from build123d import *

# Parameters (mm, degrees)
F0_W           = 430
F0_H           = 100
F1_DEPTH       = 10
F3_D           = 17.5
F4_D           = 5
F4_CBORE_D     = 11.25
F4_CBORE_DEPTH = 6
F5_D           = 6
F8_R           = 10
F9_DEPTH       = 10


with BuildPart() as f1:
    # F0 (on Front) → F1 (new body)
    with BuildSketch(Plane.XZ):
        with Locations((215, 50)):
            Rectangle(F0_W, F0_H)
    extrude(amount=F1_DEPTH)

    # F3 (through all)
    with Locations(Plane.XZ.offset(10)):
        with Locations((47.26, 57.03), (159.02, 57.03), (270.78, 57.03), (382.54, 57.03)):
            Hole(F3_D / 2)

    # F4 (through all)
    with Locations(Plane.XZ.offset(10)):
        with Locations((10, 90), (112.5, 90), (215, 90), (317.5, 90), (420, 90), (420, 10), (317.5, 10), (215, 10), (112.05, 10), (10, 10)):
            CounterBoreHole(F4_D / 2, F4_CBORE_D / 2, F4_CBORE_DEPTH)

    # F5 (through all)
    with Locations(Plane.XZ.offset(10)):
        with Locations((10, 50), (215, 50), (420, 50)):
            Hole(F5_D / 2)

    # F8 (on line) → F9 (cut)
    with BuildSketch(Plane(origin=(0, -24.8257901338, 20.831311345), x_dir=(-1, 0, 0), z_dir=(0, 0.7660444431, -0.6427876097))):
        with Locations((-16.1151010543, 22.157035768)):
            Circle(F8_R)
        with Locations((-81.1700448394, 22.157035768)):
            Circle(F8_R)
        with Locations((-175.6755411625, 22.157035768)):
            Circle(F8_R)
        with Locations((-295.1289117336, 22.157035768)):
            Circle(F8_R)
        with Locations((-396.9926536083, 22.157035768)):
            Circle(F8_R)
    extrude(amount=-F9_DEPTH, mode=Mode.SUBTRACT)


solid = f1.part
Input: part model. Units: mm. Frame: model coordinates. A direction names the side the tool comes from. Give positions to 0.01 mm unless a question says otherwise; leave off trailing zeros. Loops run counter-clockwise (first coordinate to the right, second up) from the corner with the lowest first, then second, coordinate; pieces in that order, holes last. Notation, with made-up numbers: (89, 69) -> (102, 69) arc R5 cw to (102, 77) -> close; hole circle Ø11 at (13.5, 85). An arc over 180 degrees is marked (long way). Answer as a JSON object with one key per item and string values. Group by question number.
Item 1: Pin query (flat end, axial travel): P1, Ø5.5, axis at x = 216, z = 10.5, coming from the -Y side; P2, Ø10.5, axis at x = 47.26, z = 57.03, coming from the +Y side. Return the tip coordinate at first contact, or that it passes through.
Item 2: Cut plane B-B, the plane z = 57.03. Return the cut outline in (x, y).
Item 3: Pull-direction query (X, two-part tool) for faces 3 (the flat face through (430, -5, 49)), 4 (the flat face through (216.2, -4, 87.6)), 5 (the flat face through (212, 0, 51)); classes: released by +X, released by -X, zero draft, split by the parting line, or undercut.
Item 4: Line query: probe 1 along Z at (x, y) = (420, -1.8); probe 2 along Z at (x, y) = (47.26, -7); probe 3 along X at (y, z) = (-6.75, 86). Output: solid intervals per line, ascending.
Item 5: Cut plane A-A, the plane x = 47.26. Return the cut outline in (y, z).
Item 6: Cut plane C-C, the plane x = 292.5. Return the cut outline in (y, z).
Item 7: Reachability of faces 1 (the cylindrical face through (39.177, -4.93, 53.679)), 2 (the flat face through (295.268, -7.686, 41.257)) from +Z, -Z, +X, -X, +Y, -Y: full face, straight path, thin tool, end or side. Return the list, or none.
Item 8: Cut plane D-D, the plane y = -6.75. State how many separate pieces and enclosed holes the cut face has, and give its area (3 significant figures).
Checks:
{
 "1": {"P1": "stops at y = -4", "P2": "passes through"},
 "2": {"outline": "(0, -10) -> (38.51, -10) -> (38.51, 0) -> (0, 0) -> close; (56.01, -10) -> (150.27, -10) -> (150.27, 0) -> (56.01, 0) -> close; (167.77, -10) -> (262.03, -10) -> (262.03, 0) -> (167.77, 0) -> close; (279.53, -10) -> (373.79, -10) -> (373.79, 0) -> (279.53, 0) -> close; (391.29, -10) -> (430, -10) -> (430, 0) -> (391.29, 0) -> close"},
 "3": {"face 3": "released by +X", "face 4": "undercut", "face 5": "zero draft"},
 "4": {"probe 1": "z = 0 to 7.5, 12.5 to 47, 53 to 87.5, 92.5 to 100", "probe 2": "z = 0 to 48.28, 65.78 to 100", "probe 3": "x = 0 to 6.05, 13.95 to 108.55, 116.45 to 211.05, 218.95 to 313.55, 321.45 to 416.05, 423.95 to 430"},
 "5": {"outline": "(-10, 0) -> (0, 0) -> (0, 48.28) -> (-10, 48.28) -> close; (-10, 65.78) -> (0, 65.78) -> (0, 100) -> (-10, 100) -> close"},
 "6": {"outline": "(-10, 0) -> (0, 0) -> (0, 100) -> (-10, 100) -> (-10, 49.91) -> (-4.38, 45.2) -> (-10, 38.5) -> close"},
 "7": {"face 1": "+Y, -Y", "face 2": "-Y"},
 "8": {"separate pieces": "1", "enclosed holes": "22", "area": "40,700 mm²"}
}
